Geometry: final body of the model. Coordinates: model frame, mm. Face numbers are marked on the shaded views. A direction names the side the tool comes from. Give positions to 0.01 mm unless a question says otherwise; leave off trailing zeros. Order: outer loops, then holes, each group sorted by start corner. A loop starts at its lowest first (then second) coordinate and runs counter-clockwise, first axis right, second up. Notation, with made-up numbers: (71.5, 25) - (86.5, 25) arc R14 cw to (86.5, 35) - close; hole circle Ø8 at (3.5, -11). An arc over 180 degrees is marked (long way). One line per item, written item: value.
```python
from build123d import *

# Parameters (mm, degrees)
EXTRUDE_1_DEPTH        = 14
EXTRUDE_2_DEPTH        = 7
CUT_EXTRUDE_1_DEPTH    = 38.1
CUT_EXTRUDE_2_DEPTH    = 41.028932188
HOLE_WIZARD_M4_1_D     = 4.318
HOLE_WIZARD_M4_1_DEPTH = 14
FILLET_1_R             = 5
FILLET_3_R             = 1.27
FILLET_4_R             = 1.27


with BuildPart() as part:
    # 草图1 → 凸台-拉伸1 (new body)
    with BuildSketch(Plane.XZ.offset(-1)):
        Polygon((4.743453393, -52.27499012), (35.219755662, -21.79868785), (-2.928932188, 16.35), (-41.028932188, 16.35), (-41.028932188, -16.35), align=None)
    extrude(amount=-EXTRUDE_1_DEPTH)

    # 草图2 → 凸台-拉伸2 (add)
    with BuildSketch(Plane(origin=(0, 15, 0), x_dir=(1, 0, 0), z_dir=(0, 1, 0))):
        Polygon((35.219755662, 21.79868785), (38.755289568, 18.263153944), (43.705037037, 23.212901413), (33.098435319, 33.819503131), (28.14868785, 28.869755662), align=None)
    extrude(amount=-EXTRUDE_2_DEPTH)

    # 草图3 → 切除-拉伸1 (cut)
    with BuildSketch(Plane(origin=(6.710533906, 0, 6.710533906), x_dir=(0.707106781, 0, -0.707106781), z_dir=(0.707106781, 0, 0.707106781))):
        with BuildLine():
            Line((9.538251542, 1), (30.270004579, 1))
            ThreePointArc((30.270004579, 1), (19.904128061, 10.414), (9.538251542, 1))
        make_face()
    extrude(amount=-CUT_EXTRUDE_1_DEPTH, mode=Mode.SUBTRACT)

    # 草图4 → 切除-拉伸2 (cut)
    with BuildSketch(Plane.ZY.offset(41.028932188)):
        with BuildLine():
            Line((-6.270765504, 1), (6.270765504, 1))
            ThreePointArc((6.270765504, 1), (0, 6.35), (-6.270765504, 1))
        make_face()
    extrude(amount=-CUT_EXTRUDE_2_DEPTH, mode=Mode.SUBTRACT)

    # M4 间隙孔1
    with Locations(Plane(origin=(0, 15, 0), x_dir=(1, 0, 0), z_dir=(0, 1, 0))):
        with Locations((-35.028932188, -10.35), (5, 0), (-15, 15), (-12.103043109, -10.35), (-35.028932188, 10.35), (4.743453393, 43.789708745), (26.734474288, 21.79868785)):
            Hole(HOLE_WIZARD_M4_1_D / 2, depth=HOLE_WIZARD_M4_1_DEPTH)

    # 圆角1
    fillet_1_edges = [part.edges().sort_by_distance(p)[0] for p in [
        (-41.028932188, 8, -16.35),
        (-41.028932188, 8, 16.35),
        (-2.928932188, 8, 16.35),
        (4.743453393, 8, -52.27499012),
    ]]
    fillet(fillet_1_edges, radius=FILLET_1_R)

    # 圆角3
    fillet_3_edges = [part.edges().sort_by_distance(p)[0] for p in [
        (28.14868785, 11.5, -28.869755662),
    ]]
    fillet(fillet_3_edges, radius=FILLET_3_R)

    # 圆角4
    fillet_4_edges = [part.edges().sort_by_distance(p)[0] for p in [
        (31.684221756, 8, -25.334221756),
    ]]
    fillet(fillet_4_edges, radius=FILLET_4_R)


solid = part.part
```
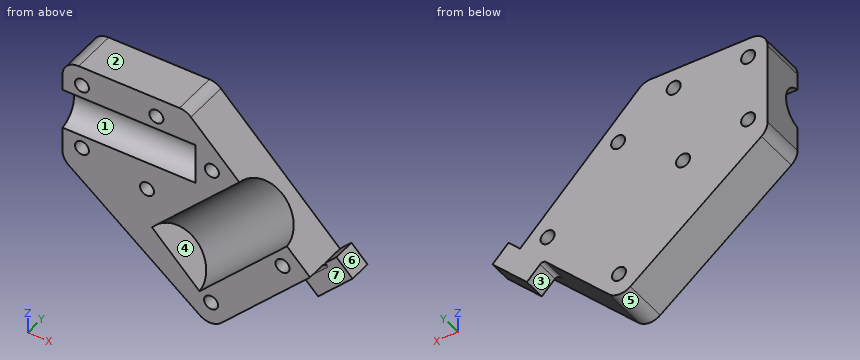
1) Material intervals for line 1 along X through (y, z) = (7.75, -15); line 2 along Z through (x, y) = (-8.5, 5.75); line 3 along X through (y, z) = (4.5, -15), sorted ascending.
Answers below:
line 1: -40.91 to -17.16, -12.84 to 3.31, 22.99 to 28.42
line 2: -41.88 to -31.96, -24.37 to -2.69, 2.69 to 16.35
line 3: -40.91 to -17.16, -12.84 to -0.13, 26.43 to 28.42
2) Section A-A, the plane y = 12.75. Return loops of the section in (x, z).
Answers below:
outline: (-41.03, -13.92) arc R5 ccw to (-39.12, -17.85) - (1.26, -49.54) arc R5 ccw to (7.88, -49.14) - (27.25, -29.77) arc R1.27 cw to (29.05, -29.77) - (33.1, -33.82) - (43.71, -23.21) - (38.76, -18.26) - (35.22, -21.8) - (-1.46, 14.89) arc R5 ccw to (-5, 16.35) - (-36.03, 16.35) arc R5 ccw to (-41.03, 11.35) - close; hole circle Ø4.32 at (-35.03, -10.35); hole circle Ø4.32 at (-35.03, 10.35); hole circle Ø4.32 at (-15, -15); hole circle Ø4.32 at (-12.1, 10.35); hole circle Ø4.32 at (4.74, -43.79); hole circle Ø4.32 at (5, 0); hole circle Ø4.32 at (26.73, -21.8)
3) Mould query, pull axis Z, two halves, no side actions, for the marked faces 4, 5, 6 and 7. Classes: released by +Z, released by -Z, zero draft, split by the parting line, or undercut.
Answers below:
face 4: undercut
face 5: released by -Z
face 6: released by +Z
face 7: zero draft
4) First-contact query: pin 1 (6 mm diameter, centred on x = 13.5, y = 7.5, fed in from -Z); pin 2 (1 mm diameter, centred on x = 12, y = 10.5, fed in from +Z); pin 3 (4 mm diameter, centred on x = -14, z = -2.5, fed in from -Y). Flat tips, straight axial feed; report the tip coordinate or a pass-through.
Answers below:
pin 1: z = -46.52
pin 2: z = 1.92
pin 3: y = 4.48
5) Section C-C, the plane x = 5. Count the separate pieces of the cut face and the enclosed holes in it, then the cut area to 3 significant figures.
Answers below:
separate pieces: 3
enclosed holes: 0
area: 494 mm^2
6) Section D-D, the plane y = 5. Return loops of the section in (x, z).
Answers below:
outline: (-41.03, -13.92) arc R5 ccw to (-39.12, -17.85) - (1.26, -49.54) arc R5 ccw to (7.88, -49.14) - (35.22, -21.8) - (27.24, -13.82) - (0.3, -40.76) - (-12.62, -27.85) - (14.33, -0.9) - (-1.46, 14.89) arc R5 ccw to (-5, 16.35) - (-36.03, 16.35) arc R5 ccw to (-41.03, 11.35) - (-41.03, 3.91) - (0, 3.91) - (0, -3.91) - (-41.03, -3.91) - close; hole circle Ø4.32 at (-35.03, -10.35); hole circle Ø4.32 at (-35.03, 10.35); hole circle Ø4.32 at (-15, -15); hole circle Ø4.32 at (-12.1, 10.35); hole circle Ø4.32 at (4.74, -43.79); hole circle Ø4.32 at (5, 0); hole circle Ø4.32 at (26.73, -21.8)
7) Section B-B, the plane z = 10.35. Return loops of the section in (x, y).
Answers below:
outline: (-41.03, 1) - (-37.19, 1) - (-37.19, 15) - (-41.03, 15) - close; (-32.87, 1) - (-14.26, 1) - (-14.26, 15) - (-32.87, 15) - close; (-9.94, 1) - (3.07, 1) - (3.07, 15) - (-9.94, 15) - close
8) Set-up query: the marked faces 1, 2 and 3. Return all of +Z, -Z, +X, -X, +Y, -Y with unobstructed straight access to the full face (end or side cutting, diameter ignored); none if empty.
Answers below:
face 1: -X, -Y
face 2: +Z, +X, -X, +Y, -Y
face 3: -Z, +Y, -Y
